```python
from build123d import *
from build123d.topology import SkipClean

# Parameters (mm, degrees)
SKETCH1_R               = 4
BOSS_EXTRUDE1_DEPTH     = 20
SKETCH2_R               = 2
BOSS_EXTRUDE2_DEPTH     = 3
CUT_EXTRUDE1_DEPTH      = 3
BOSS_EXTRUDE3_DEPTH     = 5
CUT_EXTRUDE2_DEPTH      = 101.233839294
CUT_EXTRUDE2_DEPTH_BACK = 101.233839294
BOSS_EXTRUDE4_START     = -2
BOSS_EXTRUDE4_DEPTH     = 2
CUT_EXTRUDE3_DEPTH      = 87.641828375
CUT_EXTRUDE3_DEPTH_BACK = 87.641828375
BOSS_EXTRUDE5_START     = 30
SKETCH8_R               = 4
BOSS_EXTRUDE5_DEPTH     = 30
CUT_EXTRUDE4_DEPTH      = 95.330150438
CUT_EXTRUDE4_DEPTH_BACK = 95.330150438


with BuildPart() as part:
    # Sketch1 → Boss-Extrude1 (new body)
    with BuildSketch(Plane.XY):
        with BuildLine():
            Line((0, 9), (-90, 9))
            Line((-90, 9), (-90, -9))
            Line((-90, -9), (0, -9))
            ThreePointArc((0, -9), (9, 0), (0, 9))
        make_face()
        Circle(SKETCH1_R, mode=Mode.SUBTRACT)
    extrude(amount=BOSS_EXTRUDE1_DEPTH)

    # Sketch2 → Boss-Extrude2 (add)
    with BuildSketch(Plane(origin=(0, 9, 0), x_dir=(1, 0, 0), z_dir=(0, 1, 0))):
        with Locations((-40, -10)):
            Circle(SKETCH2_R)
    extrude(amount=BOSS_EXTRUDE2_DEPTH)

    # Sketch3 → Cut-Extrude1 (cut)
    with BuildSketch(Plane(origin=(0, 9, 0), x_dir=(1, 0, 0), z_dir=(0, 1, 0))):
        with BuildLine():
            ThreePointArc((-79.971123065, -2.265451037), (-81.109001692, -1.425669976), (-81.948782753, -2.563548603))
            add(Edge.make_bspline(
                [(-75, -38.284271372), (-75.000000372, -35.299991519), (-75.743878784, -29.368041064), (-77.978217194, -20.541251955), (-80.298698299, -11.655347435), (-81.490438214, -5.604329939), (-81.948782753, -2.563548603)],
                knots=[0, 0, 0, 0, 0.171177105, 0.342354209, 0.513531314, 0.684708419, 0.684708419, 0.684708419, 0.684708419], degree=3))
            ThreePointArc((-75, -38.284271372), (-73.999999875, -39.284271247), (-73, -38.284271123))
            add(Edge.make_bspline(
                [(-73, -38.284271123), (-73.000000195, -36.723266395), (-73.196821218, -33.592705995), (-74.160174303, -27.46140767), (-76.050190168, -20.013503037), (-78.351483402, -11.19146534), (-79.520228797, -5.256805267), (-79.971123065, -2.265451037)],
                knots=[0, 0, 0, 0, 0.085588552, 0.171177105, 0.342354209, 0.513531314, 0.684708419, 0.684708419, 0.684708419, 0.684708419], degree=3))
        make_face()
    extrude(amount=-CUT_EXTRUDE1_DEPTH, mode=Mode.SUBTRACT)

    # Sketch4 → Boss-Extrude3 (add)
    with BuildSketch(Plane(origin=(0, 9, 0), x_dir=(1, 0, 0), z_dir=(0, 1, 0))):
        with BuildLine():
            Line((-90, -10), (-90, -0.41449982))
            Line((-90, -0.41449982), (-80.959952909, -0.41449982))
            ThreePointArc((-80.959952909, -0.41449982), (-79.655383082, -0.898552075), (-78.982293221, -2.116402253))
            add(Edge.make_bspline(
                [(-72, -38.284270998), (-72.000000199, -36.686938926), (-72.201891338, -33.476167151), (-73.182332484, -27.246191739), (-75.086106556, -19.748762966), (-77.377895983, -10.95977161), (-78.535124088, -5.083042932), (-78.982293221, -2.116402253)],
                knots=[0, 0, 0, 0, 0.085588552, 0.171177105, 0.342354209, 0.513531314, 0.684708419, 0.684708419, 0.684708419, 0.684708419], degree=3))
            ThreePointArc((-72, -38.284270998), (-73.99999975, -40.284271247), (-76, -38.284271497))
            add(Edge.make_bspline(
                [(-76, -38.284271497), (-76.000000181, -36.832248759), (-76.181610857, -33.942322546), (-77.093699759, -28.107055454), (-78.942441004, -20.807723253), (-80.653811295, -14.254625868), (-81.461843141, -10.616938278), (-81.594497194, -10)],
                knots=[0, 0, 0, 0, 0.085588552, 0.171177105, 0.342354209, 0.513531314, 0.548394238, 0.548394238, 0.548394238, 0.548394238], degree=3))
            Line((-81.594497194, -10), (-90, -10))
        make_face()
        with BuildLine():
            ThreePointArc((-75, -38.284271372), (-73.999999875, -39.284271247), (-73, -38.284271123))
            add(Edge.make_bspline(
                [(-73, -38.284271123), (-73.000000195, -36.723266395), (-73.196821218, -33.592705995), (-74.160174303, -27.46140767), (-76.050190168, -20.013503037), (-78.351483402, -11.19146534), (-79.520228797, -5.256805267), (-79.971123065, -2.265451037)],
                knots=[0, 0, 0, 0, 0.085588552, 0.171177105, 0.342354209, 0.513531314, 0.684708419, 0.684708419, 0.684708419, 0.684708419], degree=3))
            ThreePointArc((-79.971123065, -2.265451037), (-81.109001692, -1.425669976), (-81.948782753, -2.563548603))
            add(Edge.make_bspline(
                [(-81.948782753, -2.563548603), (-81.490438214, -5.604329939), (-80.298698299, -11.655347435), (-77.978217194, -20.541251955), (-75.743878784, -29.368041064), (-75.000000372, -35.299991519), (-75, -38.284271372)],
                knots=[0, 0, 0, 0, 0.171177105, 0.342354209, 0.513531314, 0.684708419, 0.684708419, 0.684708419, 0.684708419], degree=3))
        make_face(mode=Mode.SUBTRACT)
    extrude(amount=-BOSS_EXTRUDE3_DEPTH)

    # Sketch5 → Cut-Extrude2 (cut, two sides: drawn at the far end of the back side and taken through both)
    with BuildSketch(Plane(origin=(0, 9, 0), x_dir=(1, 0, 0), z_dir=(0, 1, 0)).offset(-CUT_EXTRUDE2_DEPTH_BACK)):
        with BuildLine():
            Line((-79.162032771, -19.999999885), (-83.13188577, -3.470019027))
            ThreePointArc((-83.13188577, -3.470019027), (-83.017493149, -1.150402786), (-81, 0))
            Line((-81, 0), (-90, 0))
            Line((-90, 0), (-90, -20))
            Line((-90, -20), (-79.162032771, -19.999999885))
        make_face()
    extrude(amount=CUT_EXTRUDE2_DEPTH + CUT_EXTRUDE2_DEPTH_BACK, mode=Mode.SUBTRACT)

    # Sketch6 → Boss-Extrude4 (add)
    with BuildSketch(Plane.XZ.offset(-4).offset(BOSS_EXTRUDE4_START)):
        with BuildLine():
            Line((-76.064161018, 20), (-78.129327832, 20))
            Line((-78.129327832, 20), (-79.162032327, 19.999999771))
            add(Edge.make_bspline(
                [(-76, 38.284271497), (-76.000000181, 36.832248759), (-76.181610857, 33.942322546), (-77.093699759, 28.107055454), (-78.268200121, 23.469809255), (-79.0949235, 20.260458438), (-79.162032327, 19.999999771)],
                knots=[0.190934795, 0.190934795, 0.190934795, 0.190934795, 0.276523348, 0.3621119, 0.533289005, 0.548394238, 0.548394238, 0.548394238, 0.548394238], degree=3))
            ThreePointArc((-76, 38.284271497), (-73.99999975, 40.284271247), (-72, 38.284270998))
            add(Edge.make_bspline(
                [(-75.031610496, 20.00000001), (-74.287622469, 22.893815084), (-73.170396852, 27.32203382), (-72.201891338, 33.476167151), (-72.000000199, 36.686938926), (-72, 38.284270998)],
                knots=[0, 0, 0, 0, 0.167009375, 0.252597927, 0.338186479, 0.338186479, 0.338186479, 0.338186479], degree=3))
            Line((-75.031610496, 20.00000001), (-76.064161018, 20))
        make_face()
    extrude(amount=BOSS_EXTRUDE4_DEPTH)

    # Sketch7 → Cut-Extrude3 (cut, two sides: drawn at the far end of the back side and taken through both)
    with BuildSketch(Plane.XY.offset(20).offset(-CUT_EXTRUDE3_DEPTH_BACK)):
        Polygon((-72, -21), (-15, -9), (-72, 4), (-92, 4), (-92, -21), align=None)
    extrude(amount=CUT_EXTRUDE3_DEPTH + CUT_EXTRUDE3_DEPTH_BACK, mode=Mode.SUBTRACT)

    # Sketch8 → Boss-Extrude5 (add)
    with SkipClean():  # the faces are left unmerged after this step: merging them gives an invalid solid
        with BuildSketch(Plane(origin=(0, 0, 0), x_dir=(-1, 0, 0), z_dir=(0, 0, -1)).offset(BOSS_EXTRUDE5_START)):
            with BuildLine():
                Line((15, -9), (72, 4))
                Line((72, 4), (81, 4))
                Line((81, 4), (81, 9))
                Line((81, 9), (0, 9))
                ThreePointArc((0, 9), (-9, 0), (0, -9))
                Line((0, -9), (15, -9))
            make_face()
            Circle(SKETCH8_R, mode=Mode.SUBTRACT)
        extrude(amount=-BOSS_EXTRUDE5_DEPTH)

    # Sketch9 → Cut-Extrude4 (cut, two sides: drawn at the far end of the back side and taken through both)
    with BuildSketch(Plane(origin=(0, 9, 0), x_dir=(1, 0, 0), z_dir=(0, 1, 0)).offset(-CUT_EXTRUDE4_DEPTH_BACK)):
        with BuildLine():
            Line((9, 0.626236109), (-26, 0.626236109))
            Line((-26, 0.626236109), (-36.200880428, -14.00000001))
            Line((-36.200880428, -14.00000001), (-76.200880428, -14.00000001))
            Line((-76.200880428, -14.00000001), (-75.031610496, -20.00000001))
            Line((-75.031610496, -20.00000001), (16, -20.00000001))
            Line((16, -20.00000001), (16, 10.626236109))
            Line((16, 10.626236109), (16, 30))
            Line((16, 30), (-81, 30))
            Line((-81, 30), (-81, 0))
            ThreePointArc((-81, 0), (-79.99562938, 0.16672565), (-78.983962224, 0.281125602))
            Line((-78.983962224, 0.281125602), (-77.857346165, -5.50000001))
            Line((-77.857346165, -5.50000001), (-40.635759862, -5.50000001))
            Line((-40.635759862, -5.50000001), (-29.388723709, 10.626236109))
            Line((-29.388723709, 10.626236109), (9, 10.626236109))
            Line((9, 10.626236109), (9, 0.626236109))
        make_face()
    extrude(amount=CUT_EXTRUDE4_DEPTH + CUT_EXTRUDE4_DEPTH_BACK, mode=Mode.SUBTRACT)

    # Mirror1: part across plane


with BuildPart() as part_1:
    add(part.part)
    add(part.part.mirror(Plane(origin=(9, -9, -10.626236109), x_dir=(1, 0, 0), z_dir=(0, 0, 1))))


solid = part_1.part
```
The listing builds one solid part. Answer for the finished solid, in the listing's coordinates (mm). A direction names the side the tool comes from. Round coordinates to 2 decimals unless told otherwise and drop trailing zeros. Loops run counter-clockwise (first coordinate to the right, second up) from the corner with the lowest first, then second, coordinate; pieces in that order, holes last. Notation, with made-up numbers: (21, 5.5) -> (70, 5.5) arc R34 ccw to (70, 35.5) -> close; hole circle Ø11 at (46, -18). An arc over 180 degrees is marked (long way). Use one line per item in the form item = value.
1. The part is cut by section C-C on x = -23. Determine the outline of the cut face in (y, z), and give its area (3 significant figures).
Answer key:
outline = (-7.18, -20.63) -> (9, -20.63) -> (9, -0.63) -> (-7.18, -0.63) -> close
area = 324 mm²
2. The part is cut by section B-B on z = -13. Determine the outline of the cut face in (x, y).
Answer key:
outline = (-31.04, -5.34) -> (-15, -9) -> (0, -9) arc R9 ccw to (0, 9) -> (-31.04, 9) -> close; hole circle Ø8 at (0, 0)
3. Find the intervals of material crossed by probe 1 along Y at (x, z) = (0, -5); probe 2 along Z at (x, y) = (-46, -1.75); probe 3 along Y at (x, z) = (-15, -16), in increasing order. Write a range as [from, to].
Answer key:
probe_1 = [-9, -4], [4, 9]
probe_2 = [-35.25, -26.75], [5.5, 14]
probe_3 = [-9, 9]
4. The part is cut by section A-A on x = -1.5. Determine the outline of the cut face in (y, z).
Answer key:
outline = (-9, -20.63) -> (-3.71, -20.63) -> (-3.71, -0.63) -> (-9, -0.63) -> close; (3.71, -20.63) -> (9, -20.63) -> (9, -0.63) -> (3.71, -0.63) -> close
5. A tool of negligible diameter and unlimited length cuts with its end or side. For faces 4 (the flat face through (-35.09, 1.54, -18.8)), 5 (the flat face through (-77, 6, 20)), 6 (the flat face through (-75.624, 6.465, -38.21)), from which of +Z, -Z, +X, -X, +Y, -Y can it reach the whole face along a straight path? Write none if from no direction.
Answer key:
face_4 = +Y, -Y
face_5 = +Y
face_6 = +X, +Y, -Y
6. Flat-ended cylindrical pins translate along their axes: pin 1 Ø8 at (x, y) = (-59, 5) entering from -Z; pin 2 Ø9 at (x, z) = (-78, 16) entering from -Y; pin 3 Ø4 at (y, z) = (8.5, 28.5) entering from -X. Find the tip coordinate at first contact, or state that the pin passes through.
Answer key:
pin_1 = -35.25
pin_2 = 4
pin_3 = -77.55
7. For a pull along Z with two mould halves and no side action, classify faces 1 (the flat face through (-8, 0, -0.626)), 2 (the flat face through (-8, 0, -20.626)), 3 (the cylindrical face through (-83.035, 6.465, 1.179)) as released by +Z, released by -Z, zero draft, split by the parting line, or undercut.
Answer key:
face_1 = released by +Z
face_2 = released by -Z
face_3 = undercut
